Autodesk Inventor part; units mm, degrees
ref_plane "YZ Plane" through (0, 0, 0) normal (1, 0, 0) x (0, 1, 0)
ref_plane "XZ Plane" through (0, 0, 0) normal (0, 1, 0) x (-1, 0, 0)
ref_plane "XY Plane" through (0, 0, 0) normal (0, 0, 1) x (1, 0, 0)
sketch "Sketch1" plane through (0, 0, 0) normal (0, 0, 1) x (1, 0, 0)
  arc A0 (15, 17) -> (-15, 17) centre (0, 17) ccw
  line L0 (20, 17) -> (20, 0)
  line L1 (-20, 17) -> (-20, 0)
  line L2 (30, 5) -> (30, 0)
  line L3 (30, 0) -> (-30, 0)
  line L4 (-30, 0) -> (-30, 5)
  line L5 (15, 17) -> (15, 0)
  line L6 (-15, 17) -> (-15, 0)
  arc A1 (20, 17) -> (-20, 17) centre (0, 17) ccw
  line L7 (-30, 5) -> (-20, 5)
  line L8 (20, 5) -> (30, 5)
  point P0 (0, 0)
  point P1 (0, 0)
  dimension "d0" = 30
  dimension "d1" = 17
  dimension "d3" = 60
  dimension "d5" = 20
  dimension "d6" = 5
  dimension "d7" = 5
extrude "Extrusion1" add sketch "Sketch1" along normal blind 10 contours A0 L6 L3 L1 A1 L0 L5 | L0 L8 L2 L3 | L3 L4 L7 L1
hole "Hole1" at (25, 5, 5) direction (0, -1, 0) diameter 6 end through all
hole "Hole2" at (-25, 5, 5) direction (0, -1, 0) diameter 6 end through all
properties part number "holder"
Part model, mm, in its own coordinate system. A direction names the side the tool comes from. Coordinates: 2 decimals unless noted, no trailing zeros. Write each loop counter-clockwise with the first axis right and the second up, starting at its lowest first coordinate (ties: lowest second). Pieces come first, ordered by that corner, then holes.
Item 1: Slice it at B-B (y = 10). Write the cut outline in (x, z).
Item 2: Mould opens along X. For faces 5 (the face through (26.8, 2.5, 2.6)), 6 (the face through (0, 37, 5)), 7 (the face through (15.4, 15.8, 10)) say: released by +X, released by -X, zero draft, split by the parting line, or undercut.
Item 3: Slice it at A-A (z = 5). Write the cut outline in (x, y), and give its area (3 significant figures).
Item 4: Probe line 1 (X direction, y = 3.1, z = 5); line 2 (Z direction, x = -25, y = 2); line 3 (X direction, y = 6, z = 8.75). List the from-to ranges inside material, lowest first.
Item 5: Slice it at C-C (x = 25). Write the cut outline in (y, z).
Item 6: Pin check, flat tips, straight feed: pin 1 (6 mm diameter, centred on y = 24, z = 9, fed in from -X); pin 2 (5 mm diameter, centred on x = -24, z = 4.5, fed in from +Y); pin 3 (3 mm diameter, centred on x = -10, z = 5, fed in from +Y). Stop position of each tip, or through.
Item 7: Which spindle directions (+Z, -Z, +X, -X, +Y, -Y) get a long thin tool onto all of the face, cutting with end or side? Do faces 1 (the face through (15.4, 15.8, 0)), 2 (the face through (22.7, 5, 2.7)), 3 (the face through (-27.3, 5, 2.7)), 4 (the face through (-15, 9, 5)). Say none if no direction does.
Item 8: Slice it at D-D (z = 1.25). Write the cut outline in (x, y), and give its area (3 significant figures).
Results found:
1. outline: (-20, 0) - (-15, 0) - (-15, 10) - (-20, 10) - close; (15, 0) - (20, 0) - (20, 10) - (15, 10) - close
2. face 5: undercut
2. face 6: split by the parting line
2. face 7: zero draft
3. outline: (-30, 0) - (-28, 0) - (-28, 5) - (-30, 5) - close; (-22, 0) - (-15, 0) - (-15, 17) arc R15 cw to (15, 17) - (15, 0) - (22, 0) - (22, 5) - (20, 5) - (20, 17) arc R20 ccw to (-20, 17) - (-20, 5) - (-22, 5) - close; (28, 0) - (30, 0) - (30, 5) - (28, 5) - close
3. area: 485 mm2
4. line 1: x = -30 to -28, -22 to -15, 15 to 22, 28 to 30
4. line 2: z = 0 to 2, 8 to 10
4. line 3: x = -20 to -15, 15 to 20
5. outline: (0, 0) - (5, 0) - (5, 2) - (0, 2) - close; (0, 8) - (5, 8) - (5, 10) - (0, 10) - close
6. pin 1: stops at x = -19.6
6. pin 2: stops at y = 5
6. pin 3: stops at y = 35.1
7. face 1: -Z, +X, -X, +Y, -Y
7. face 2: +Z, -Z, +X, +Y
7. face 3: +Z, -Z, -X, +Y
7. face 4: +Z, -Z, -Y
8. outline: (-30, 0) - (-15, 0) - (-15, 17) arc R15 cw to (15, 17) - (15, 0) - (30, 0) - (30, 5) - (20, 5) - (20, 17) arc R20 ccw to (-20, 17) - (-20, 5) - (-30, 5) - close
8. area: 545 mm2
